```python
from build123d import *

# Parameters (mm, degrees)
PAD_DEPTH       = 54
SKETCH001_R     = 1.6
POCKET_DEPTH    = 6
SKETCH002_R     = 6.1
POCKET001_DEPTH = 5
FILLET_R        = 4
FILLET001_R     = 4
FILLET002_R     = 4
FILLET003_R     = 4
CHAMFER_SIZE    = 0.4
CHAMFER001_SIZE = 0.4
CHAMFER002_SIZE = 0.4
CHAMFER003_SIZE = 0.4


with BuildPart() as part:
    # Sketch → Pad (new body)
    with BuildSketch(Plane.XY):
        Polygon((0, 0), (0, 6), (9, 6), (9, 40), (53, 40), (53, 6), (62, 6), (62, 0), (49, 0), (49, 36), (13, 36), (13, 0), align=None)
    extrude(amount=PAD_DEPTH)

    # Sketch001 (on Face8 of Pad) → Pocket (cut)
    with BuildSketch(Plane.XZ):
        with Locations((5, 5)):
            Circle(SKETCH001_R)
        with Locations((57, 5)):
            Circle(SKETCH001_R)
        with Locations((57, 49)):
            Circle(SKETCH001_R)
        with Locations((5, 49)):
            Circle(SKETCH001_R)
    extrude(amount=-POCKET_DEPTH, mode=Mode.SUBTRACT)

    # Sketch002 (on Face10 of Pocket) → Pocket001 (cut)
    with BuildSketch(Plane(origin=(0, 40, 0), x_dir=(-1, 0, 0), z_dir=(0, 1, 0))):
        with Locations((-31, 26)):
            Circle(SKETCH002_R)
    extrude(amount=-POCKET001_DEPTH, mode=Mode.SUBTRACT)

    # Fillet
    fillet_edges = [part.edges().sort_by_distance(p)[0] for p in [
        (62, 3, 0),
        (62, 3, 54),
        (0, 3, 54),
        (0, 3, 0),
    ]]
    fillet(fillet_edges, radius=FILLET_R)

    # Fillet001
    fillet001_edges = [part.edges().sort_by_distance(p)[0] for p in [
        (53, 40, 27),
        (9, 40, 27),
    ]]
    fillet(fillet001_edges, radius=FILLET001_R)

    # Fillet002
    fillet002_edges = [part.edges().sort_by_distance(p)[0] for p in [
        (49, 0, 27),
        (13, 0, 27),
    ]]
    fillet(fillet002_edges, radius=FILLET002_R)

    # Fillet003
    fillet003_edges = [part.edges().sort_by_distance(p)[0] for p in [
        (49, 36, 27),
        (13, 36, 27),
    ]]
    fillet(fillet003_edges, radius=FILLET003_R)

    # Chamfer
    chamfer_edges = [part.edges().sort_by_distance(p)[0] for p in [
        (37.1, 40, 26),
    ]]
    chamfer(chamfer_edges, length=CHAMFER_SIZE)

    # Chamfer001
    chamfer001_edges = [part.edges().sort_by_distance(p)[0] for p in [
        (55.4, 6, 5),
        (55.4, 6, 49),
        (3.4, 6, 5),
        (3.4, 6, 49),
    ]]
    chamfer(chamfer001_edges, length=CHAMFER001_SIZE)

    # Chamfer002
    chamfer002_edges = [part.edges().sort_by_distance(p)[0] for p in [
        (37.1, 36, 26),
    ]]
    chamfer(chamfer002_edges, length=CHAMFER002_SIZE)

    # Chamfer003
    chamfer003_edges = [part.edges().sort_by_distance(p)[0] for p in [
        (3.4, 0, 49),
        (3.4, 0, 5),
        (55.4, 0, 49),
        (55.4, 0, 5),
    ]]
    chamfer(chamfer003_edges, length=CHAMFER003_SIZE)


solid = part.part
```
Here's how the part is built. I have some questions about the finished solid (model axes, mm). A direction names the side the tool comes from. Round coordinates to 2 decimals unless told otherwise and drop trailing zeros. Write each loop counter-clockwise with the first axis right and the second up, starting at its lowest first coordinate (ties: lowest second). Pieces come first, ordered by that corner, then holes.
Q1. Which directions (+Z, -Z, +X, -X, +Y, -Y) give clear straight access to the entire face, cutting with the end or side of a thin tool? Please do faces 5 (the flat face through (9, 21, 27)), 6 (the flat face through (49, 18, 27)), 7 (the cylindrical face through (58.48, 2.96, 4.39)).
Q2. If we section it at A-A on z = 26: Write out the boundary of the cut face in (x, y), plus the area to 3 significant figures.
Q3. Will these pins go through, and if not, where does the flat tip stop? P1, Ø14, axis at y = 21.5, z = 37.5, coming from the +X side; P2, Ø9, axis at y = 14.5, z = 20, coming from the -X side; P3, Ø22.5, axis at y = 17, z = 27.5, coming from the -X side; P4, Ø3, axis at x = 18, z = 40.5, coming from the -Y side.
Q4. Please list where these lines run through material, in increasing order: probe 1 along X at (y, z) = (25.5, 23.5); probe 2 along X at (y, z) = (5.5, 43.5); probe 3 along Z at (x, y) = (57, 4.55).
Q5. If we section it at C-C on y = 23.5: Write out the boundary of the cut face in (x, z).
Q6. If we mould it in two halves opening along X, with no side actions, what happens to faces 1 (the cylindrical face through (58.526, 2.964, 49.481)), 2 (the flat face through (31, 40, 33)), 3 (the cylindrical face through (10.141, 38.797, 27.378)), 4 (the flat face through (53, 21, 27))? For each: +X half, -X half, draft (parallel to the pull), parting line (faces both ways), or undercut.
Q7. If we section it at B-B on x = 31: Write out the boundary of the cut face in (y, z).
Q8. If we section it at D-D on x = 57: Write out the boundary of the cut face in (y, z).
Answer below:
1. face 5: +Z, -Z, -X, +Y
1. face 6: +Z, -Z, -Y
1. face 7: +Y, -Y
2. outline: (0, 0) - (9, 0) arc R4 ccw to (13, 4) - (13, 32) arc R4 cw to (17, 36) - (24.5, 36) - (24.9, 36.4) - (24.9, 39.6) - (24.5, 40) - (13, 40) arc R4 ccw to (9, 36) - (9, 6) - (0, 6) - close; (37.1, 36.4) - (37.5, 36) - (45, 36) arc R4 cw to (49, 32) - (49, 4) arc R4 ccw to (53, 0) - (62, 0) - (62, 6) - (53, 6) - (53, 36) arc R4 ccw to (49, 40) - (37.5, 40) - (37.1, 39.6) - close
2. area: 516 mm2
3. P1: stops at x = 53
3. P2: stops at x = 9
3. P3: stops at x = 0
3. P4: stops at y = 35.97
4. probe 1: x = 9 to 13, 49 to 53
4. probe 2: x = 0 to 13, 49 to 62
4. probe 3: z = 0 to 3.4, 6.6 to 47.4, 50.6 to 54
5. outline: (9, 0) - (13, 0) - (13, 54) - (9, 54) - close; (49, 0) - (53, 0) - (53, 54) - (49, 54) - close
6. face 1: undercut
6. face 2: draft
6. face 3: -X half
6. face 4: +X half
7. outline: (36, 0) - (40, 0) - (40, 19.5) - (39.6, 19.9) - (36.4, 19.9) - (36, 19.5) - close; (36, 32.5) - (36.4, 32.1) - (39.6, 32.1) - (40, 32.5) - (40, 54) - (36, 54) - close
8. outline: (0, 0) - (6, 0) - (6, 3) - (5.6, 3.4) - (0.4, 3.4) - (0, 3) - close; (0, 7) - (0.4, 6.6) - (5.6, 6.6) - (6, 7) - (6, 47) - (5.6, 47.4) - (0.4, 47.4) - (0, 47) - close; (0, 51) - (0.4, 50.6) - (5.6, 50.6) - (6, 51) - (6, 54) - (0, 54) - close
